from build123d import *

# Parameters (mm, degrees)
SKETCH1_W           = 5
SKETCH1_H           = 1.25
BOSS_EXTRUDE1_DEPTH = 7.3
SKETCH3_W           = 1.25
SKETCH3_H           = 5
BOSS_EXTRUDE2_DEPTH = 3.5
SKETCH4_W           = 2.5
SKETCH4_H           = 5
BOSS_EXTRUDE3_DEPTH = 14
BOSS_EXTRUDE4_DEPTH = 8
SKETCH6_R           = 1.49705526
BOSS_EXTRUDE5_DEPTH = 1
SKETCH7_R           = 1.25
BOSS_EXTRUDE6_DEPTH = 8
SKETCH8_R           = 1.49705526
BOSS_EXTRUDE7_DEPTH = 1
FILLET2_R           = 1.5


with BuildPart() as part:
    # Sketch1 → Boss-Extrude1 (new body)
    with BuildSketch(Plane(origin=(0, 0, 0), x_dir=(0, 0, -1), z_dir=(1, 0, 0))):
        with Locations((0.720440882, 1.136523046)):
            Rectangle(SKETCH1_W, SKETCH1_H)
    extrude(amount=BOSS_EXTRUDE1_DEPTH)

    # Sketch3 → Boss-Extrude2 (add)
    with BuildSketch(Plane(origin=(0, 1.761523046, 0), x_dir=(1, 0, 0), z_dir=(0, 1, 0))):
        with Locations((0.625, 0.720440882)):
            Rectangle(SKETCH3_W, SKETCH3_H)
    extrude(amount=BOSS_EXTRUDE2_DEPTH)

    # Sketch4 → Boss-Extrude3 (add)
    with BuildSketch(Plane(origin=(0, 1.761523046, 0), x_dir=(1, 0, 0), z_dir=(0, 1, 0))):
        with Locations((6.05, 0.720440882)):
            Rectangle(SKETCH4_W, SKETCH4_H)
    extrude(amount=BOSS_EXTRUDE3_DEPTH)

    # Sketch5 → Boss-Extrude4 (add)
    with BuildSketch(Plane(origin=(0, 0, -3.220440882), x_dir=(-1, 0, 0), z_dir=(0, 0, -1))):
        with BuildLine():
            ThreePointArc((-4.8, 14.511523046), (-5.166116524, 15.395406523), (-6.05, 15.761523046))
            ThreePointArc((-6.05, 15.761523046), (-6.52835429, 15.666372462), (-6.933883476, 15.395406523))
            Line((-6.933883476, 15.395406523), (-5.166116524, 13.62763957))
            ThreePointArc((-5.166116524, 13.62763957), (-4.895150584, 14.033168756), (-4.8, 14.511523046))
        make_face()
        with BuildLine():
            ThreePointArc((-6.933883476, 15.395406523), (-7.20484942, 14.989877325), (-7.3, 14.511523021))
            ThreePointArc((-7.3, 14.511523021), (-6.933883468, 13.627639561), (-6.05, 13.261523046))
            ThreePointArc((-6.05, 13.261523046), (-5.57164571, 13.35667363), (-5.166116524, 13.62763957))
            Line((-5.166116524, 13.62763957), (-6.933883476, 15.395406523))
        make_face()
    extrude(amount=BOSS_EXTRUDE4_DEPTH)

    # Sketch6 → Boss-Extrude5 (add)
    with BuildSketch(Plane(origin=(0, 0, -11.220440882), x_dir=(-1, 0, 0), z_dir=(0, 0, -1))):
        with Locations((-6.05, 14.511523046)):
            Circle(SKETCH6_R)
    extrude(amount=BOSS_EXTRUDE5_DEPTH)

    # Sketch7 → Boss-Extrude6 (add)
    with BuildSketch(Plane.XY.offset(1.779559118)):
        with Locations((6.05, 14.511523046)):
            Circle(SKETCH7_R)
    extrude(amount=BOSS_EXTRUDE6_DEPTH)

    # Sketch8 → Boss-Extrude7 (add)
    with BuildSketch(Plane.XY.offset(9.779559118)):
        with Locations((6.05, 14.511523046)):
            Circle(SKETCH8_R)
    extrude(amount=BOSS_EXTRUDE7_DEPTH)

    # Fillet2
    fillet2_edges = [part.edges().sort_by_distance(p)[0] for p in [
        (0, 0.511523046, -0.720440882),
    ]]
    fillet(fillet2_edges, radius=FILLET2_R)


solid = part.part
Source: CAD feature listing. Evaluate the final solid. Frame: model axes, mm. A direction names the side the tool comes from. Give positions to 0.01 mm unless a question says otherwise; leave off trailing zeros. Write each loop counter-clockwise with the first axis right and the second up, starting at its lowest first coordinate (ties: lowest second). Pieces come first, ordered by that corner, then holes. Notation, with made-up numbers: (60.5, 62) -> (77.5, 62) arc R20 ccw to (77.5, 85) -> close; hole circle Ø5 at (-1, 53). An arc over 180 degrees is marked (long way). Return JSON: item names as keys, results as strings. Group by question number.
1. Mould query, pull axis Z, two halves, no side actions, for faces 5 (the face through (7.042, 15.504, 1.78)), 6 (the face through (6, 15, -12.22)), 7 (the face through (0, 4, -1)). Classes: +Z half, -Z half, draft (parallel to the pull), parting line (faces both ways), or undercut.
2. Access query for faces 1 (the face through (3, 1.762, -1)), 2 (the face through (1, 5.262, -1)), 3 (the face through (5.05, 15.5, 1.78)), 4 (the face through (6, 15.762, -1)). Directions: +Z, -Z, +X, -X, +Y, -Y. A direction counts if a zero-diameter tool reaches every point of the face in a straight line with its end or side. Return the directions, or none.
3. Material intervals for line 1 (Z direction, x = 5, y = 13.5); line 2 (Z direction, x = 4.75, y = 14.5); line 3 (Y direction, x = 3, z = -0.5), sorted ascending. Write a range as from..to.
4. Section B-B, the plane z = -7.5. Output: boundary loops of the cut face in (x, y).
5. Section D-D, the plane y = 10. Output: boundary loops of the cut face in (x, z), then the cut area to 3 significant figures.
6. Section C-C, the plane x = 5.5. Output: boundary loops of the cut face in (y, z), then the cut area to 3 significant figures.
7. Pin query (flat end, axial travel): pin 1 Ø3 at (x, z) = (6, 0) entering from +Y; pin 2 Ø1 at (x, z) = (5, 5) entering from +Y; pin 3 Ø2 at (x, y) = (5.5, 10) entering from -Z; pin 4 Ø1.5 at (x, y) = (4, 5) entering from -Z. Return the tip coordinate at first contact, or that it passes through.
8. Section A-A, the plane y = 4.5. Output: boundary loops of the cut face in (x, z), then the cut area to 4 significant figures.
Determined:
{
 "1": {"face 5": "undercut", "face 6": "-Z half", "face 7": "draft"},
 "2": {"face 1": "+Z, -Z, +Y", "face 2": "+Z, -Z, -X, +Y", "face 3": "-X, +Y", "face 4": "+X, -X, +Y"},
 "3": {"line 1": "z = -12.22..-11.22, -3.22..1.78, 9.78..10.78", "line 2": "z = -12.22..-11.22, 9.78..10.78", "line 3": "y = 0.51..1.76"},
 "4": {"outline": "circle Ø2.5 at (6.05, 14.51)"},
 "5": {"outline": "(4.8, -3.22) -> (7.3, -3.22) -> (7.3, 1.78) -> (4.8, 1.78) -> close", "area": "12.5 mm2"},
 "6": {"outline": "(0.51, -3.22) -> (13.39, -3.22) -> (13.39, -11.22) -> (13.12, -11.22) -> (13.12, -12.22) -> (15.9, -12.22) -> (15.9, -11.22) -> (15.63, -11.22) -> (15.63, -3.22) -> (15.76, -3.22) -> (15.76, 1.78) -> (15.63, 1.78) -> (15.63, 9.78) -> (15.9, 9.78) -> (15.9, 10.78) -> (13.12, 10.78) -> (13.12, 9.78) -> (13.39, 9.78) -> (13.39, 1.78) -> (0.51, 1.78) -> close", "area": "118 mm2"},
 "7": {"pin 1": "stops at y = 15.76", "pin 2": "stops at y = 15.63", "pin 3": "stops at z = -3.22", "pin 4": "passes through"},
 "8": {"outline": "(0, -3.22) -> (1.25, -3.22) -> (1.25, 1.78) -> (0, 1.78) -> close; (4.8, -3.22) -> (7.3, -3.22) -> (7.3, 1.78) -> (4.8, 1.78) -> close", "area": "18.75 mm2"}
}
